Input: part model. Units: mm. Frame: model coordinates. A direction names the side the tool comes from. Coordinates: 2 decimals unless noted, no trailing zeros. Loops run counter-clockwise (first coordinate to the right, second up) from the corner with the lowest first, then second, coordinate; pieces in that order, holes last. Notation, with made-up numbers: M 7,31.5 L 31,31.5 A20 cw 31,61.5 Z; hole C 25.25,-36 d6. An arc over 180 degrees is marked long. Use a Markdown table: item, result. Add a question column.
1. Set-up query: faces 1 (the flat face through (25, 26, 0)), 2 (the flat face through (17, 23.109, 4)). Return all of +Z, -Z, +X, -X, +Y, -Y with unobstructed straight access to the full face (end or side cutting, diameter ignored); none if empty.
2. Line query: L1, parallel to Y at x = 36, z = 1.5 (3 decimals); L2, parallel to X at y = 40, z = 2; L3, parallel to Y at x = 42.5, z = 3.5. Output: solid intervals per line, ascending. Write a range as [from, to].
3. Section D-D on y = 46.5. Output: boundary loops of the cut face in (x, z), then the cut area to 3 significant figures.
4. Section A-A on y = 39.37. Output: boundary loops of the cut face in (x, z), then the cut area to 3 significant figures.
5. Draft query along X for faces 3 (the flat face through (0, 25, 4)), 4 (the flat face through (25, 0, 4)), 5 (the flat face through (25, 26, 1.27)). Return one class per face: +X half, -X half, draft (parallel to the pull), parting line (faces both ways), or undercut.
6. Section C-C on y = 20. Output: boundary loops of the cut face in (x, z), then the cut area to 3 significant figures.
7. Section B-B on x = 42. Output: boundary loops of the cut face in (y, z).
```python
from build123d import *

# Parameters (mm, degrees)
F0_W       = 50.8
F0_H       = 50.8
F1_DEPTH   = 7.62
F2_T       = -1.27
F3_W       = 1.27
F3_H       = 43.18
F4_DEPTH   = 6.35
F5_R       = 1.27
F6_DEPTH   = 25.4
F7_W       = 12.7
F7_H       = 1.27
F8_DEPTH   = 6.35
F9_R       = 1.27
F10_DEPTH  = 25.4
F11_W      = 15.24
F11_H      = 1.27
F11_W_2    = 17.78
F12_DEPTH  = 6.35
F13_W      = 35.56
F13_H      = 1.279007
F13_R      = 1.27
F14_DEPTH  = 6.35
F14_FACE_R = 1.27
F15_DEPTH  = 25.4


with BuildPart() as f1:
    # F0 (on Top) → F1 (new body)
    with BuildSketch(Plane.XY):
        with Locations((25.4, 25.4)):
            Rectangle(F0_W, F0_H)
    extrude(amount=F1_DEPTH)

    # F2
    f2_openings = [f1.faces().sort_by_distance(p)[0] for p in [
        (25.4, 25.4, 7.62),
    ]]
    offset(amount=F2_T, openings=f2_openings)

    # F3 (on face) → F4 (join)
    with BuildSketch(Plane.XY.offset(1.27)):
        with Locations((6.985, 22.86)):
            Rectangle(F3_W, F3_H)
    extrude(amount=F4_DEPTH)

    # F5 (on face) → F6 (cut)
    with BuildSketch(Plane.XY.offset(1.27)):
        with Locations((3.532713, 9.804559)):
            Circle(F5_R)
        with Locations((3.532713, 4.248444)):
            Circle(F5_R)
    extrude(amount=-F6_DEPTH, mode=Mode.SUBTRACT)

    # F7 (on face) → F8 (join)
    with BuildSketch(Plane.XY.offset(1.27)):
        with Locations((13.97, 43.815)):
            Rectangle(F7_W, F7_H)
        Polygon((21.59, 44.45), (20.32, 44.45), (20.32, 43.18), (20.32, 35.56), (21.59, 35.56), align=None)
        Polygon((21.59, 35.56), (20.32, 35.56), (11.43, 35.56), (11.43, 34.29), (21.59, 34.29), align=None)
    extrude(amount=F8_DEPTH)

    # F9 (on face) → F10 (cut)
    with BuildSketch(Plane.XY.offset(1.27)):
        with Locations((17.22843, 39.37)):
            Circle(F9_R)
    extrude(amount=-F10_DEPTH, mode=Mode.SUBTRACT)

    # F11 (on face) → F12 (join)
    with BuildSketch(Plane.XY.offset(1.27)):
        with Locations((36.5252, 43.815)):
            Rectangle(F11_W, F11_H)
        Polygon((44.1452, 44.45), (44.1452, 43.18), (44.1452, 19.05), (45.4152, 19.05), (45.4152, 44.45), align=None)
        Polygon((45.4152, 19.05), (44.1452, 19.05), (7.62, 19.05), (7.62, 17.78), (45.4152, 17.78), align=None)
        with Locations((16.51, 23.743602)):
            Rectangle(F11_W_2, F11_H)
        Polygon((25.4, 34.538602), (25.4, 24.378602), (25.4, 23.108602), (26.67, 23.108602), (26.67, 34.538602), align=None)
    extrude(amount=F12_DEPTH)

    # F13 (on face) → F14 (join)
    with BuildSketch(Plane.XY.offset(1.27)):
        Polygon((13.97, 12.436993), (13.97, 13.716), (12.7, 13.716), (12.7, 5.715), (13.97, 5.715), align=None)
        with Locations((31.75, 13.076496)):
            Rectangle(F13_W, F13_H)
        Polygon((13.97, 5.715), (12.7, 5.715), (12.7, 4.445), (38.1, 4.445), (38.1, 5.715), align=None)
        with Locations((17.586783, 9.075997)):
            Circle(F13_R)
    extrude(amount=F14_DEPTH)

    # F14_face (on face) → F15 (cut)
    with BuildSketch(Plane(origin=(17.586783, 9.075997, 7.62), x_dir=(1, 0, 0), z_dir=(0, 0, 1))):
        Circle(F14_FACE_R)
    extrude(amount=-F15_DEPTH, mode=Mode.SUBTRACT)


solid = f1.part
```
Answers below:
| question | item | result |
|---|---|---|
| 1 | face 1 | -Z, +X, -X, +Y, -Y |
| 1 | face 2 | +Z |
| 2 | L1 | y = [0, 1.27], [4.445, 5.715], [12.437, 13.716], [17.78, 19.05], [43.18, 44.45], [49.53, 50.8] |
| 2 | L2 | x = [0, 1.27], [6.35, 7.62], [20.32, 21.59], [44.15, 45.42], [49.53, 50.8] |
| 2 | L3 | y = [0, 1.27], [12.44, 13.72], [17.78, 19.05], [43.18, 44.45], [49.53, 50.8] |
| 3 | outline | M 0,0 L 50.8,0 L 50.8,7.62 L 49.53,7.62 L 49.53,1.27 L 1.27,1.27 L 1.27,7.62 L 0,7.62 Z |
| 3 | area | 80.6 mm² |
| 4 | outline | M 0,0 L 15.96,0 L 15.96,1.27 L 7.62,1.27 L 7.62,7.62 L 6.35,7.62 L 6.35,1.27 L 1.27,1.27 L 1.27,7.62 L 0,7.62 Z; M 18.5,0 L 50.8,0 L 50.8,7.62 L 49.53,7.62 L 49.53,1.27 L 45.42,1.27 L 45.42,7.62 L 44.15,7.62 L 44.15,1.27 L 21.59,1.27 L 21.59,7.62 L 20.32,7.62 L 20.32,1.27 L 18.5,1.27 Z |
| 4 | area | 102 mm² |
| 5 | face 3 | -X half |
| 5 | face 4 | draft |
| 5 | face 5 | undercut |
| 6 | outline | M 0,0 L 50.8,0 L 50.8,7.62 L 49.53,7.62 L 49.53,1.27 L 45.42,1.27 L 45.42,7.62 L 44.15,7.62 L 44.15,1.27 L 7.62,1.27 L 7.62,7.62 L 6.35,7.62 L 6.35,1.27 L 1.27,1.27 L 1.27,7.62 L 0,7.62 Z |
| 6 | area | 96.8 mm² |
| 7 | outline | M 0,0 L 50.8,0 L 50.8,7.62 L 49.53,7.62 L 49.53,1.27 L 44.45,1.27 L 44.45,7.62 L 43.18,7.62 L 43.18,1.27 L 19.05,1.27 L 19.05,7.62 L 17.78,7.62 L 17.78,1.27 L 13.72,1.27 L 13.72,7.62 L 12.44,7.62 L 12.44,1.27 L 1.27,1.27 L 1.27,7.62 L 0,7.62 Z |
